Geometry check sheet. Reference: drawing and pictorial views, mm from the part's lowest x, y, z. Give positions to 0.01 mm unless a question says otherwise; leave off trailing zeros. Order: outer loops, then holes, each group sorted by start corner. A loop starts at its lowest first (then second) coordinate and runs counter-clockwise, first axis right, second up. Notation, with made-up numbers: (-36.75, -28) - (15.25, -28) arc R19 ccw to (15.25, 1) - close; hole circle Ø5 at (-13, -19.5). An arc over 180 degrees is marked (long way). Answer in a Markdown table with one row per item.
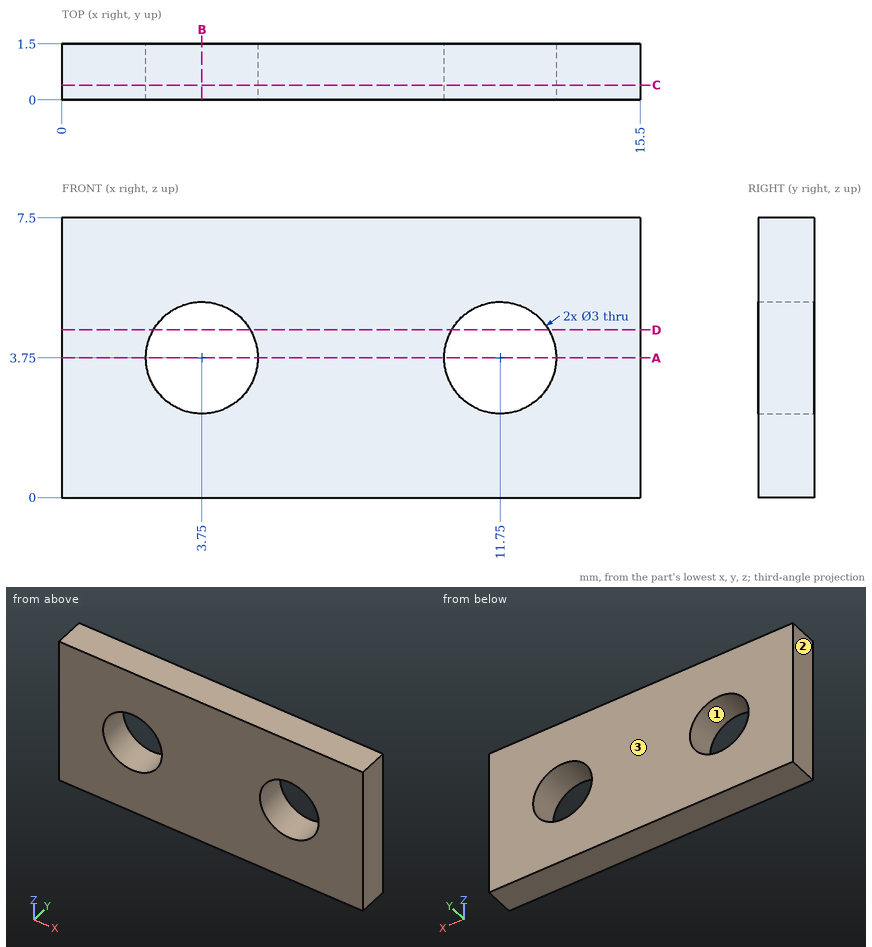
(1) Mould release check, pull along X, two halves, no side actions. Record for the marked faces 1, 2 and 3: pulls with the +X half, pulls with the -X half, needs draft (parallel to the pull), parting line crosses it, or undercut.
Geometry says:
| item | result |
|---|---|
| face 1 | undercut |
| face 2 | pulls with the -X half |
| face 3 | needs draft |
(2) Thickness scan on L1, parallel to X at y = 1.25, z = 3.75; L2, parallel to Z at x = 11.75, y = 0.9; L3, parallel to X at y = 1.3, z = 4.5. Record the ranges inside material, lowest first.
Geometry says:
| item | result |
|---|---|
| L1 | 0 to 2.25, 5.25 to 10.25, 13.25 to 15.5 |
| L2 | 0 to 2.25, 5.25 to 7.5 |
| L3 | 0 to 2.45, 5.05 to 10.45, 13.05 to 15.5 |
(3) Cross-section at D-D, the plane z = 4.5. Record the cut outline in (x, y), then the cut area to 3 significant figures.
Geometry says:
| item | result |
|---|---|
| outline | (0, 0) - (2.45, 0) - (2.45, 1.5) - (0, 1.5) - close; (5.05, 0) - (10.45, 0) - (10.45, 1.5) - (5.05, 1.5) - close; (13.05, 0) - (15.5, 0) - (15.5, 1.5) - (13.05, 1.5) - close |
| area | 15.5 mm² |
(4) Cross-section at A-A, the plane z = 3.75. Record the cut outline in (x, y).
Geometry says:
| item | result |
|---|---|
| outline | (0, 0) - (2.25, 0) - (2.25, 1.5) - (0, 1.5) - close; (5.25, 0) - (10.25, 0) - (10.25, 1.5) - (5.25, 1.5) - close; (13.25, 0) - (15.5, 0) - (15.5, 1.5) - (13.25, 1.5) - close |
(5) Cross-section at C-C, the plane y = 0.4. Record the cut outline in (x, z).
Geometry says:
| item | result |
|---|---|
| outline | (0, 0) - (15.5, 0) - (15.5, 7.5) - (0, 7.5) - close; hole circle Ø3 at (3.75, 3.75); hole circle Ø3 at (11.75, 3.75) |
(6) Cross-section at B-B, the plane x = 3.75. Record the cut outline in (y, z).
Geometry says:
| item | result |
|---|---|
| outline | (0, 0) - (1.5, 0) - (1.5, 2.25) - (0, 2.25) - close; (0, 5.25) - (1.5, 5.25) - (1.5, 7.5) - (0, 7.5) - close |
